```python
from build123d import *

# Parameters (mm, degrees)
F0_W           = 101.2207046151
F0_H           = 84.5743343234
F0_W_2         = 95.3139290214
F0_H_2         = 79.7415152192
F1_DEPTH       = 12.7
F2_W           = 95.3139290214
F2_H           = 80.278493464
F3_DEPTH       = 2.032
F5_D           = 4.572
F5_CBORE_D     = 4.572
F5_CBORE_DEPTH = 4.572


with BuildPart() as f1:
    # F0 (on Top) → F1 (new body)
    with BuildSketch(Plane.XY):
        Rectangle(F0_W, F0_H)
        Rectangle(F0_W_2, F0_H_2, mode=Mode.SUBTRACT)
    extrude(amount=F1_DEPTH)

    # F2 (on Top) → F3 (join)
    with BuildSketch(Plane.XY):
        Rectangle(F2_W, F2_H)
    extrude(amount=F3_DEPTH)

    # F5 (through all)
    with Locations(Plane(origin=(0, 0, 0), x_dir=(1, 0, 0), z_dir=(0, 0, -1))):
        with Locations((0, -36.6952344775)):
            CounterBoreHole(F5_D / 2, F5_CBORE_D / 2, F5_CBORE_DEPTH)


solid = f1.part
```
Geometry check sheet. Reference: the model listing, model coordinates, mm. A direction names the side the tool comes from. Coordinates: 2 decimals unless noted, no trailing zeros. Loops run counter-clockwise (first coordinate to the right, second up) from the corner with the lowest first, then second, coordinate; pieces in that order, holes last.
Item 1: Sectioned sample at B-B, the plane z = 5. Record the boundary of the cut face in (x, y).
Item 2: Go/stop test with flat-tipped pins: pin 1 Ø4 at (x, y) = (0, 36.7) entering from +Z; pin 2 Ø5 at (x, y) = (2, -5.5) entering from +Z. Record where each tip stops, or that it passes through.
Item 3: Sectioned sample at A-A, the plane x = 0. Record the boundary of the cut face in (y, z).
Item 4: Release check for a two-part mould opening along Y. For faces 1 (the face through (-1, -42.287, 6)), 2 (the face through (-4, -41, 12.7)), 3 (the face through (-1, 1, 2.032)) record: released by +Y, released by -Y, zero draft, split by the parting line, or undercut.
Item 5: Access from +Z, -Z, +X, -X, +Y, -Y to the whole of each face (thin tool, end or side, straight path). Record for faces 4 (the face through (0.3, 34.43, 1.03)), 5 (the face through (-47.657, -1, 7)).
Item 6: Sectioned sample at C-C, the plane y = 28. Record the boundary of the cut face in (x, z).
Item 7: Thickness scan on line 1 (Y direction, x = 0, z = 0.8); line 2 (X direction, y = -13, z = 5.75); line 3 (Y direction, x = -28.5, z = 9). Record the ranges inside material, lowest first.
Check result:
1. outline: (-50.61, -42.29) - (50.61, -42.29) - (50.61, 42.29) - (-50.61, 42.29) - close; hole (-47.66, -39.87) - (47.66, -39.87) - (47.66, 39.87) - (-47.66, 39.87) - close
2. pin 1: passes through
2. pin 2: stops at z = 2.03
3. outline: (-42.29, 0) - (34.41, 0) - (34.41, 2.03) - (-39.87, 2.03) - (-39.87, 12.7) - (-42.29, 12.7) - close; (38.98, 0) - (42.29, 0) - (42.29, 12.7) - (39.87, 12.7) - (39.87, 2.03) - (38.98, 2.03) - close
4. face 1: released by -Y
4. face 2: zero draft
4. face 3: undercut
5. face 4: +Z, -Z
5. face 5: +Z
6. outline: (-50.61, 0) - (50.61, 0) - (50.61, 12.7) - (47.66, 12.7) - (47.66, 2.03) - (-47.66, 2.03) - (-47.66, 12.7) - (-50.61, 12.7) - close
7. line 1: y = -42.29 to 34.41, 38.98 to 42.29
7. line 2: x = -50.61 to -47.66, 47.66 to 50.61
7. line 3: y = -42.29 to -39.87, 39.87 to 42.29
